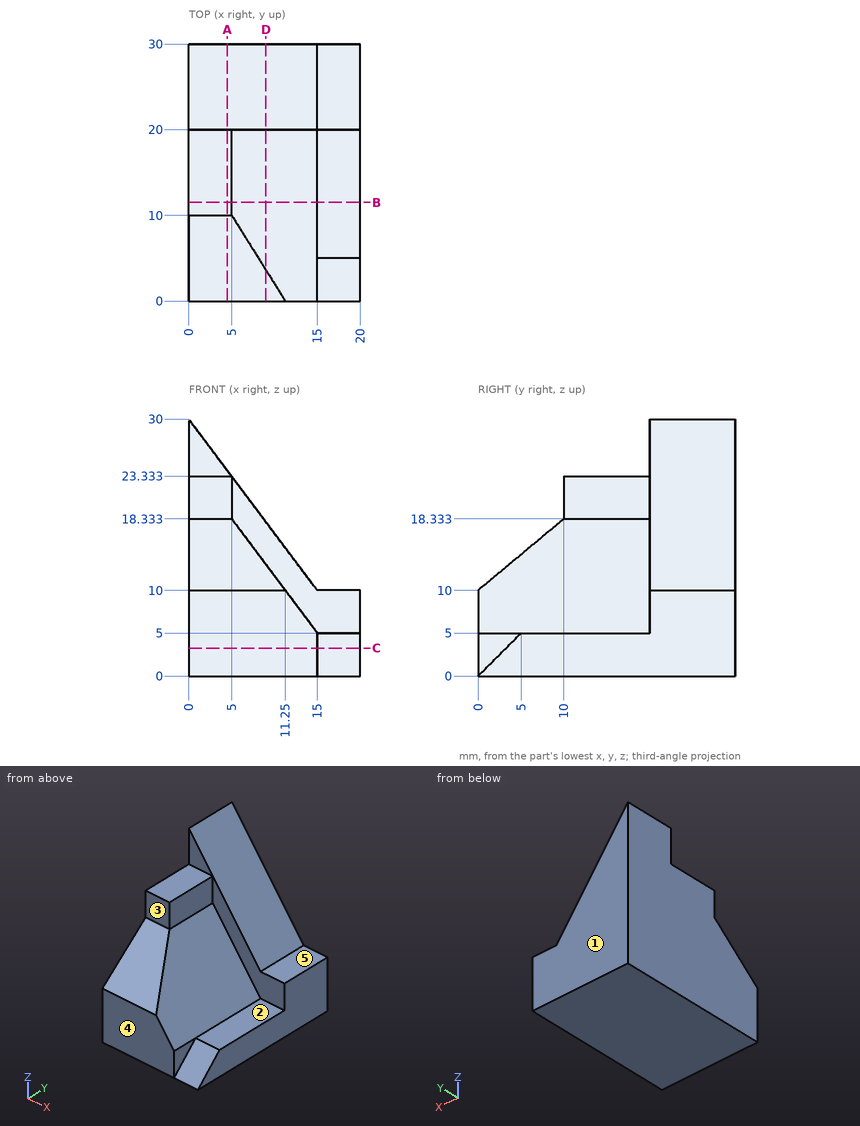
Input: dimensioned drawing with shaded views. Units: mm. Origin: part minimum x, y, z. A direction names the side the tool comes from. Coordinates: 2 decimals unless noted, no trailing zeros. Order: outer loops, then holes, each group sorted by start corner. A loop starts at its lowest first (then second) coordinate and runs counter-clockwise, first axis right, second up. Notation, with made-up numbers: M 12,37.5 L 57,37.5 A12 cw 57,51.5 Z; hole C -36,42 d10. An arc over 180 degrees is marked long. Answer as CSV lines item,"result".
Q1. Section D-D on x = 9. Return the cut outline in (y, z).
Answers:
outline,"M 0,0 L 30,0 L 30,18 L 20,18 L 20,13 L 3.6,13 L 0,10 Z"
Q2. Section A-A on x = 4.5. Return the cut outline in (y, z), and give its area (3 significant figures).
Answers:
outline,"M 0,0 L 30,0 L 30,24 L 20,24 L 20,23.33 L 10,23.33 L 10,18.33 L 0,10 Z"
area,"615 mm^2"
Q3. Section C-C on z = 3.25. Return the cut outline in (x, y).
Answers:
outline,"M 0,0 L 15,0 L 15,3.25 L 20,3.25 L 20,30 L 0,30 Z"
Q4. Set-up query: the marked faces 1, 2, 3, 4 and 5. Return all of +Z, -Z, +X, -X, +Y, -Y with unobstructed straight access to the full face (end or side cutting, diameter ignored); none if empty.
Answers:
face 1,"+Z, -Z, +X, -X, +Y"
face 2,"+Z, +X, -Y"
face 3,"+Z, +X, -X, -Y"
face 4,"+Z, -Z, +X, -X, -Y"
face 5,"+Z, +X, +Y, -Y"
Q5. Section B-B on y = 11.5. Return the cut outline in (x, z), and give its area (3 significant figures).
Answers:
outline,"M 0,0 L 20,0 L 20,5 L 15,5 L 5,18.33 L 5,23.33 L 0,23.33 Z"
area,"258 mm^2"
Q6. First-contact query: P1, Ø2.5, axis at y = 17, z = 19.5, coming from the +X side; P2, Ø2.5, axis at x = 18.5, y = 27, coming from the +Z side; P3, Ø6, axis at x = 15, y = 7, coming from the +Z side. Flat tips, straight axial feed; report the tip coordinate or a pass-through.
Answers:
P1,"stops at x = 5.06"
P2,"stops at z = 10"
P3,"stops at z = 9"
Q7. Line query: probe 1 along Z at (x, y) = (15.75, 16.5); probe 2 along X at (y, z) = (23.5, 15); probe 3 along Z at (x, y) = (19, 21.75). Output: solid intervals per line, ascending. Write a range as [from, to].
Answers:
probe 1,"z = [0, 5]"
probe 2,"x = [0, 11.25]"
probe 3,"z = [0, 10]"
